Model file for the job. Use its own axes, mm. A direction names the side the tool comes from. Coordinates: 2 decimals unless noted, no trailing zeros. Loops run counter-clockwise (first coordinate to the right, second up) from the corner with the lowest first, then second, coordinate; pieces in that order, holes last.
from build123d import *

# Parameters (mm, degrees)
SKETCH2_W             = 28.575
SKETCH2_H             = 152.4
BOSS_EXTRUDE1_DEPTH   = 9.525
F_3_0MM_DOWEL_HOLE1_D = 3
LPATTERN1_COUNT       = 4
LPATTERN1_PITCH       = 42.333333333
SKETCH12_R            = 2.05
CUT_EXTRUDE1_DEPTH    = 156.348048749
SKETCH12_4_R          = 10.975
CUT_EXTRUDE2_DEPTH    = 4
SKETCH15_R            = 2.5
CUT_EXTRUDE3_DEPTH    = 156.154169296
SKETCH13_R            = 2.6
CUT_EXTRUDE4_DEPTH    = 156.348048749
SKETCH17_W            = 41.28
SKETCH17_H            = 9.525
CUT_EXTRUDE5_DEPTH    = 8.575


with BuildPart() as part:
    # Sketch2 → Boss-Extrude1 (new body)
    with BuildSketch(Plane(origin=(0, 0, 0), x_dir=(1, 0, 0), z_dir=(0, 1, 0))):
        with Locations((14.2875, 76.2)):
            Rectangle(SKETCH2_W, SKETCH2_H)
    extrude(amount=BOSS_EXTRUDE1_DEPTH)

    # Ø3.0mm Dowel Hole1 (through all)
    with Locations(Plane.ZY):
        with Locations((-139.7, 4.7625)):
            f_3_0mm_dowel_hole1 = Hole(F_3_0MM_DOWEL_HOLE1_D / 2)

    # LPattern1: Ø3.0mm Dowel Hole1 ×4, 1 skipped
    with Locations(*[(0, 0, i * LPATTERN1_PITCH) for i in range(1, LPATTERN1_COUNT) if i not in (2,)]):
        add(f_3_0mm_dowel_hole1, mode=Mode.SUBTRACT)

    # Sketch12 → Cut-Extrude1 (cut, through all)
    with BuildSketch(Plane(origin=(0, 9.525, 0), x_dir=(1, 0, 0), z_dir=(0, 1, 0))):
        with Locations(Location((14.2875, 120.65, 0), (0, 0, 270))):
            Circle(SKETCH12_R)
    extrude(amount=-CUT_EXTRUDE1_DEPTH, mode=Mode.SUBTRACT)

    # Sketch12<4> → Cut-Extrude2 (cut)
    with BuildSketch(Plane(origin=(0, 9.525, 0), x_dir=(1, 0, 0), z_dir=(0, 1, 0))):
        with Locations(Location((14.2875, 31.75, 0), (0, 0, 270))):
            Circle(SKETCH12_4_R)
    extrude(amount=-CUT_EXTRUDE2_DEPTH, mode=Mode.SUBTRACT)

    # Sketch15 → Cut-Extrude3 (cut, through all)
    with BuildSketch(Plane(origin=(0, 5.525, 0), x_dir=(1, 0, 0), z_dir=(0, 1, 0))):
        with Locations(Location((14.2875, 31.75, 0), (0, 0, 270))):
            Circle(SKETCH15_R)
    extrude(amount=-CUT_EXTRUDE3_DEPTH, mode=Mode.SUBTRACT)

    # Sketch13 → Cut-Extrude4 (cut, through all)
    with BuildSketch(Plane.ZY):
        with Locations((-80, 4.7625)):
            Circle(SKETCH13_R)
        with Locations((-47.79, 4.7625)):
            Circle(SKETCH13_R)
    extrude(amount=-CUT_EXTRUDE4_DEPTH, mode=Mode.SUBTRACT)

    # Sketch17 → Cut-Extrude5 (cut)
    with BuildSketch(Plane.ZY):
        with Locations((-63.895, 4.7625)):
            Rectangle(SKETCH17_W, SKETCH17_H)
    extrude(amount=-CUT_EXTRUDE5_DEPTH, mode=Mode.SUBTRACT)


solid = part.part
Q1. Slice it at B-B (x = 21.75). List the corners of the cut face in (y, z) (1 decimal), and give its area (3 significant figures).
Answers:
outline: (0, -152.4) - (9.5, -152.4) - (9.5, -39.8) - (5.5, -39.8) - (5.5, -23.7) - (9.5, -23.7) - (9.5, 0) - (0, 0) - close; hole circle Ø5.2 at (4.8, -80); hole circle Ø5.2 at (4.8, -47.8); hole circle Ø3 at (4.8, -139.7); hole circle Ø3 at (4.8, -97.4); hole circle Ø3 at (4.8, -12.7)
area: 1,320 mm2
Q2. Mould opens along Y. For faces 1 (the cylindrical face through (18.435, 3.18, -49.853)), 2 (the cylindrical face through (14.488, 3.85, -96.176)), 3 (the flat face through (4, 5, -84.535)), 4 (the flat face through (14, 9.525, -77)) say: +Y half, -Y half, draft (parallel to the pull), parting line (faces both ways), or undercut.
Answers:
face 1: undercut
face 2: undercut
face 3: draft
face 4: +Y half
Q3. Flat gauge pins, fed straight in: P1, Ø3.5, axis at x = 14.29, z = -120.65, coming from the +Y side; P2, Ø3, axis at y = 7.5, z = -72.5, coming from the -X side (3 decimals). Where does each tip first touch, or does it go through?
Answers:
P1: passes through
P2: stops at x = 8.575
Q4. Which spindle directions (+Z, -Z, +X, -X, +Y, -Y) get a long thin tool onto all of the face, cutting with end or side? Do faces 5 (the cylindrical face through (4.55, 7.55, -26.69)), 6 (the flat face through (14, 0, -77)), 7 (the flat face through (4, 5, -43.255)). Say none if no direction does.
Answers:
face 5: +Y
face 6: +Z, -Z, +X, -X, -Y
face 7: -X, +Y, -Y
Q5. Slice it at C-C (z = -120.65). List the corners of the cut face in (x, y) (1 decimal).
Answers:
outline: (0, 0) - (12.2, 0) - (12.2, 9.5) - (0, 9.5) - close; (16.3, 0) - (28.6, 0) - (28.6, 9.5) - (16.3, 9.5) - close
Q6. Drill centre lines: line 1 (Z direction, x = 22, y = 5); line 2 (Z direction, x = 8.25, y = 1.75) (3 decimals); line 3 (Z direction, x = 13.5, y = 8.25). Where is each one in solid material? Low to high.
Answers:
line 1: z = -152.4 to -141.18, -138.22 to -98.85, -95.89 to -82.59, -77.41 to -50.38, -45.2 to -14.18, -11.22 to 0
line 2: z = -152.4 to -84.535, -43.255 to 0
line 3: z = -152.4 to -122.54, -118.76 to -42.7, -20.8 to 0
Q7. Slice it at A-A (z = -12.7). List the corners of the cut face in (x, y) (1 decimal).
Answers:
outline: (0, 0) - (28.6, 0) - (28.6, 3.3) - (0, 3.3) - close; (0, 6.3) - (28.6, 6.3) - (28.6, 9.5) - (0, 9.5) - close
Q8. Slice it at D-D (z = -62). List the corners of the cut face in (x, y) (3 decimals), and give its area (4 significant figures).
Answers:
outline: (8.575, 0) - (28.575, 0) - (28.575, 9.525) - (8.575, 9.525) - close
area: 190.5 mm2
